Could you check a few things on this model? Use its own coordinates, in mm. Face numbers are marked on the shaded views. A direction names the side the tool comes from. Coordinates: 2 decimals unless noted, no trailing zeros. Write each loop counter-clockwise with the first axis right and the second up, starting at its lowest first coordinate (ties: lowest second). Pieces come first, ordered by that corner, then holes.
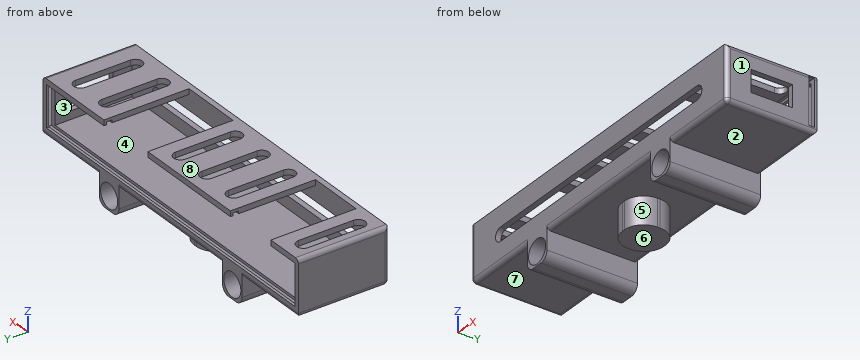
```python
from build123d import *

# Parameters (mm, degrees)
ESBO_O1_W                = 130
ESBO_O1_H                = 33
RESSALTO_EXTRUS_O1_DEPTH = 3
ESBO_O2_W                = 130
ESBO_O2_H                = 33
ESBO_O2_W_2              = 126
ESBO_O2_H_2              = 29
EXTRUS_O_FINA1_DEPTH     = 17
ESBO_O3_W                = 126.5
ESBO_O3_H                = 15
CORTE_EXTRUS_O1_DEPTH    = 2
ESBO_O4_W                = 8
ESBO_O4_H                = 15
CORTE_EXTRUS_O2_DEPTH    = 2
ESBO_O7_W                = 42
ESBO_O7_H                = 2
ESBO_O7_W_2              = 12
ESBO_O7_W_3              = 29
RESSALTO_EXTRUS_O2_DEPTH = 29
ESBO_O8_W                = 20.6
ESBO_O8_H                = 2
ESBO_O8_W_2              = 22.4
CORTE_EXTRUS_O4_DEPTH    = 2
CORTE_EXTRUS_O3_REACH    = 134.56
ESBO_O5_W                = 17
ESBO_O5_H                = 2
CORTE_EXTRUS_O5_DEPTH    = 2
CORTE_EXTRUS_O6_DEPTH    = 2
ESBO_O11_W               = 10
ESBO_O11_H               = 33
RESSALTO_EXTRUS_O3_DEPTH = 10
ESBO_O12_R               = 4.35
CORTE_EXTRUS_O7_DEPTH    = 76.591004756
ESBO_O13_W               = 15
ESBO_O13_H               = 15
RESSALTO_EXTRUS_O4_DEPTH = 10
FILETE1_R                = 7
FILETE2_R                = 3
FILETE3_R                = 1.5


with BuildPart() as part:
    # Esboço1 → Ressalto-extrusão1 (new body)
    with BuildSketch(Plane.XY):
        Rectangle(ESBO_O1_W, ESBO_O1_H)
    extrude(amount=RESSALTO_EXTRUS_O1_DEPTH)

    # Esboço2 → Extrusão-Fina1 (add)
    with BuildSketch(Plane.XY.offset(3)):
        Rectangle(ESBO_O2_W, ESBO_O2_H)
        Rectangle(ESBO_O2_W_2, ESBO_O2_H_2, mode=Mode.SUBTRACT)
    extrude(amount=EXTRUS_O_FINA1_DEPTH)

    # Esboço3 → Corte-extrusão1 (cut)
    with BuildSketch(Plane(origin=(0, 16.5, 0), x_dir=(1, 0, 0), z_dir=(0, 1, 0))):
        with Locations((0, -10.5)):
            Rectangle(ESBO_O3_W, ESBO_O3_H)
    extrude(amount=-CORTE_EXTRUS_O1_DEPTH, mode=Mode.SUBTRACT)

    # Esboço4 → Corte-extrusão2 (cut)
    with BuildSketch(Plane(origin=(65, 0, 0), x_dir=(0, 0, -1), z_dir=(1, 0, 0))):
        with Locations((-10, 0)):
            Rectangle(ESBO_O4_W, ESBO_O4_H)
    extrude(amount=-CORTE_EXTRUS_O2_DEPTH, mode=Mode.SUBTRACT)

    # Esboço7 → Ressalto-extrusão2 (add)
    with BuildSketch(Plane(origin=(0, -14.5, 0), x_dir=(1, 0, 0), z_dir=(0, 1, 0))):
        with Locations((-9.4, -19)):
            Rectangle(ESBO_O7_W, ESBO_O7_H)
        with Locations((-57, -19)):
            Rectangle(ESBO_O7_W_2, ESBO_O7_H)
        with Locations((48.5, -19)):
            Rectangle(ESBO_O7_W_3, ESBO_O7_H)
    extrude(amount=RESSALTO_EXTRUS_O2_DEPTH)

    # Esboço8 → Corte-extrusão4 (cut)
    with BuildSketch(Plane(origin=(0, 16.5, 0), x_dir=(1, 0, 0), z_dir=(0, 1, 0))):
        with Locations((-40.7, -19)):
            Rectangle(ESBO_O8_W, ESBO_O8_H)
        with Locations((22.8, -19)):
            Rectangle(ESBO_O8_W_2, ESBO_O8_H)
    extrude(amount=-CORTE_EXTRUS_O4_DEPTH, mode=Mode.SUBTRACT)

    # Corte-extrusão3: up to this face of the body (flat: up to its plane)
    corte_extrus_o3_end = Plane(part.part.faces().sort_by_distance((-63.25, 15.5, 10.5))[0])
    # Esboço5 → Corte-extrusão3 (cut, up to the picked face)
    with BuildSketch(Plane(origin=(65, 0, 0), x_dir=(0, 0, -1), z_dir=(1, 0, 0)), mode=Mode.PRIVATE) as corte_extrus_o3_sk1:
        with Locations((-10.5, 14.5)):
            Rectangle(ESBO_O5_W, ESBO_O5_H)
    corte_extrus_o3_tool1 = split(extrude(corte_extrus_o3_sk1.sketch, amount=-CORTE_EXTRUS_O3_REACH, mode=Mode.PRIVATE), bisect_by=corte_extrus_o3_end, keep=Keep.BOTH, mode=Mode.PRIVATE)
    add(corte_extrus_o3_tool1.solids().sort_by(Axis((65, 14.5, 10.5), (-1, 0, 0)))[0], mode=Mode.SUBTRACT)

    # Esboço9 → Corte-extrusão5 (cut)
    with BuildSketch(Plane.XY.offset(20)):
        with BuildLine():
            Line((-61, -10), (-61, 10))
            ThreePointArc((-61, 10), (-58.5, 12.5), (-56, 10))
            Line((-56, 10), (-56, -10))
            ThreePointArc((-56, -10), (-58.5, -12.5), (-61, -10))
        make_face()
        with BuildLine():
            Line((-25.4, -10), (-25.4, 10))
            ThreePointArc((-25.4, 10), (-22.9, 12.5), (-20.4, 10))
            Line((-20.4, 10), (-20.4, -10))
            ThreePointArc((-20.4, -10), (-22.9, -12.5), (-25.4, -10))
        make_face()
        with BuildLine():
            Line((-11.9, -10), (-11.9, 10))
            ThreePointArc((-11.9, 10), (-9.4, 12.5), (-6.9, 10))
            Line((-6.9, 10), (-6.9, -10))
            ThreePointArc((-6.9, -10), (-9.4, -12.5), (-11.9, -10))
        make_face()
        with BuildLine():
            Line((1.6, -10), (1.6, 10))
            ThreePointArc((1.6, 10), (4.1, 12.5), (6.6, 10))
            Line((6.6, 10), (6.6, -10))
            ThreePointArc((6.6, -10), (4.1, -12.5), (1.6, -10))
        make_face()
        with BuildLine():
            Line((39, -10), (39, 10))
            ThreePointArc((39, 10), (41.5, 12.5), (44, 10))
            Line((44, 10), (44, -10))
            ThreePointArc((44, -10), (41.5, -12.5), (39, -10))
        make_face()
        with BuildLine():
            Line((52.5, -10), (52.5, 10))
            ThreePointArc((52.5, 10), (55, 12.5), (57.5, 10))
            Line((57.5, 10), (57.5, -10))
            ThreePointArc((57.5, -10), (55, -12.5), (52.5, -10))
        make_face()
    extrude(amount=-CORTE_EXTRUS_O5_DEPTH, mode=Mode.SUBTRACT)

    # Esboço10 → Corte-extrusão6 (cut)
    with BuildSketch(Plane.XZ.offset(16.5)):
        with BuildLine():
            Line((-50, 12.5), (50, 12.5))
            ThreePointArc((50, 12.5), (52.5, 10), (50, 7.5))
            Line((50, 7.5), (-50, 7.5))
            ThreePointArc((-50, 7.5), (-52.5, 10), (-50, 12.5))
        make_face()
    extrude(amount=-CORTE_EXTRUS_O6_DEPTH, mode=Mode.SUBTRACT)

    # Esboço11 → Ressalto-extrusão3 (add)
    with BuildSketch(Plane(origin=(0, 0, 0), x_dir=(-1, 0, 0), z_dir=(0, 0, -1))):
        with Locations((-31.35, 0)):
            Rectangle(ESBO_O11_W, ESBO_O11_H)
        with Locations((31.35, 0)):
            Rectangle(ESBO_O11_W, ESBO_O11_H)
    extrude(amount=RESSALTO_EXTRUS_O3_DEPTH)

    # Esboço12 → Corte-extrusão7 (cut, through all)
    with BuildSketch(Plane.XZ.offset(16.5)):
        with Locations(Location((-31.35, -5, 0), (0, 0, 270))):
            Circle(ESBO_O12_R)
        with Locations(Location((31.35, -5, 0), (0, 0, 90))):
            Circle(ESBO_O12_R)
    extrude(amount=-CORTE_EXTRUS_O7_DEPTH, mode=Mode.SUBTRACT)

    # Esboço13 → Ressalto-extrusão4 (add)
    with BuildSketch(Plane(origin=(0, 0, 0), x_dir=(-1, 0, 0), z_dir=(0, 0, -1))):
        Rectangle(ESBO_O13_W, ESBO_O13_H)
    extrude(amount=RESSALTO_EXTRUS_O4_DEPTH)

    # Filete1
    filete1_edges = [part.edges().sort_by_distance(p)[0] for p in [
        (-7.5, -7.5, -5),
        (-7.5, 7.5, -5),
        (7.5, 7.5, -5),
        (7.5, -7.5, -5),
    ]]
    fillet(filete1_edges, radius=FILETE1_R)

    # Filete2
    filete2_edges = [part.edges().sort_by_distance(p)[0] for p in [
        (26.35, 0, -10),
        (36.35, 0, -10),
        (-36.35, 0, -10),
        (-26.35, 0, -10),
    ]]
    fillet(filete2_edges, radius=FILETE2_R)

    # Filete3
    # the kernel refuses this fillet: 1.5 mm, written as the material it takes off along each edge
    with BuildSketch(Plane(origin=(63.5, -15, 1.5), x_dir=(0, -1, 0), z_dir=(1, 0, 0))) as filete3_piece_1_section:
        Polygon((0, 0), (FILETE3_R, 0), (FILETE3_R, FILETE3_R), (0, FILETE3_R), align=None)
    filete3_piece_1 = extrude(amount=FILETE3_R, mode=Mode.PRIVATE)
    filete3_piece_1 = filete3_piece_1 - Plane(origin=(63.5, -15, 1.5), x_dir=(0, 0.7071067811865475, 0.7071067811865475), z_dir=(1, 0, 0)) * Sphere(FILETE3_R, mode=Mode.PRIVATE)
    add(filete3_piece_1, mode=Mode.SUBTRACT)
    with BuildSketch(Plane(origin=(-63.5, -15, 1.5), x_dir=(0, -1, 0), z_dir=(-1, 0, 0))) as filete3_piece_2_section:
        Polygon((0, 0), (FILETE3_R, 0), (FILETE3_R, -FILETE3_R), (0, -FILETE3_R), align=None)
    filete3_piece_2 = extrude(amount=FILETE3_R, mode=Mode.PRIVATE)
    filete3_piece_2 = filete3_piece_2 - Plane(origin=(-63.5, -15, 1.5), x_dir=(0, 0.7071067811865475, 0.7071067811865475), z_dir=(-1, 0, 0)) * Sphere(FILETE3_R, mode=Mode.PRIVATE)
    add(filete3_piece_2, mode=Mode.SUBTRACT)
    with BuildSketch(Plane(origin=(68.75, 16.5, 0), x_dir=(0, 0, 1), z_dir=(-1, 0, 0)), Plane(origin=(-36.35, 16.5, 0), x_dir=(0, 0, 1), z_dir=(-1, 0, 0))) as filete3_piece_3:
        with BuildLine():
            CenterArc((FILETE3_R, -FILETE3_R), FILETE3_R, 90, 90)
            Line((0, -FILETE3_R), (0, 0))
            Line((0, 0), (FILETE3_R, 0))
        make_face()
    extrude(amount=32.4, mode=Mode.SUBTRACT)
    with BuildSketch(Plane(origin=(26.35, 16.5, 0), x_dir=(0, 0, 1), z_dir=(-1, 0, 0))) as filete3_piece_4:
        with BuildLine():
            CenterArc((FILETE3_R, -FILETE3_R), FILETE3_R, 90, 90)
            Line((0, -FILETE3_R), (0, 0))
            Line((0, 0), (FILETE3_R, 0))
        make_face()
    extrude(amount=52.7, mode=Mode.SUBTRACT)
    with BuildSketch(Plane(origin=(65, -15, 0), x_dir=(-1, 0, 0), z_dir=(0, 1, 0)), Plane(origin=(-65, 20.25, 0), x_dir=(1, 0, 0), z_dir=(0, -1, 0))) as filete3_piece_5:
        with BuildLine():
            CenterArc((FILETE3_R, FILETE3_R), FILETE3_R, 180, 90)
            Line((0, FILETE3_R), (0, 0))
            Line((0, 0), (FILETE3_R, 0))
        make_face()
    extrude(amount=35.25, mode=Mode.SUBTRACT)
    with BuildSketch(Plane(origin=(65, -16.5, 1.5), x_dir=(-1, 0, 0), z_dir=(0, 0, 1)), Plane(origin=(-65, -16.5, 23.75), x_dir=(1, 0, 0), z_dir=(0, 0, -1))) as filete3_piece_6:
        with BuildLine():
            CenterArc((FILETE3_R, -FILETE3_R), FILETE3_R, 90, 90)
            Line((0, -FILETE3_R), (0, 0))
            Line((0, 0), (FILETE3_R, 0))
        make_face()
    extrude(amount=22.25, mode=Mode.SUBTRACT)
    with BuildSketch(Plane(origin=(65, -20.25, 20), x_dir=(0, 0, -1), z_dir=(0, 1, 0))) as filete3_piece_7:
        with BuildLine():
            CenterArc((FILETE3_R, FILETE3_R), FILETE3_R, 180, 90)
            Line((0, FILETE3_R), (0, 0))
            Line((0, 0), (FILETE3_R, 0))
        make_face()
    extrude(amount=40.5, mode=Mode.SUBTRACT)
    with BuildSketch(Plane(origin=(-65, 20.25, 20), x_dir=(1, 0, 0), z_dir=(0, -1, 0))) as filete3_piece_8:
        with BuildLine():
            CenterArc((FILETE3_R, -FILETE3_R), FILETE3_R, 90, 90)
            Line((0, -FILETE3_R), (0, 0))
            Line((0, 0), (FILETE3_R, 0))
        make_face()
    extrude(amount=40.5, mode=Mode.SUBTRACT)
    with BuildSketch(Plane(origin=(36.35, -16.5, 0), x_dir=(0, 0, 1), z_dir=(1, 0, 0)), Plane(origin=(-63.5, -16.5, 0), x_dir=(0, 0, 1), z_dir=(1, 0, 0))) as filete3_piece_9:
        with BuildLine():
            CenterArc((FILETE3_R, -FILETE3_R), FILETE3_R, 90, 90)
            Line((0, -FILETE3_R), (0, 0))
            Line((0, 0), (FILETE3_R, 0))
        make_face()
    extrude(amount=27.15, mode=Mode.SUBTRACT)
    with BuildSketch(Plane(origin=(-26.35, -16.5, 0), x_dir=(0, 1, 0), z_dir=(1, 0, 0))) as filete3_piece_10:
        with BuildLine():
            CenterArc((FILETE3_R, FILETE3_R), FILETE3_R, 180, 90)
            Line((0, FILETE3_R), (0, 0))
            Line((0, 0), (FILETE3_R, 0))
        make_face()
    extrude(amount=52.7, mode=Mode.SUBTRACT)


solid = part.part
```
1. Please list where these lines run through material, in increasing order: line 1 along Z through (x, y) = (-31, -2); line 2 along X through (y, z) = (-0.5, -5); line 3 along X through (y, z) = (-0.5, 15).
Verdict:
line 1: z = -10 to -9.34, -0.66 to 3
line 2: x = -36.35 to -35.7, -27 to -26.35, -7.5 to 7.5, 26.35 to 27, 35.7 to 36.35
line 3: x = -65 to -63, 63 to 65
2. On a 3-axis mill with a long thin cutter (end or side, diameter ignored), from which of +Z, -Z, +X, -X, +Y, -Y can I reach the whole of each face in a straight line? I mean the marked faces 4, 5, 6, 7 and 8. Say none if no direction works.
Verdict:
face 4: +Y
face 5: -Z, -Y
face 6: -Z, +X, -X, +Y, -Y
face 7: -Z, -X, +Y, -Y
face 8: +Z, +X, -X, +Y, -Y
3. I want a section at A-A on x = 31.35. Please give me the cut outline in (y, z), plus the area to 3 significant figures.
Verdict:
outline: (-16.5, -10) - (16.5, -10) - (16.5, -9.35) - (-16.5, -9.35) - close; (-16.5, -0.65) - (16.5, -0.65) - (16.5, 3) - (15.5, 3) - (15.5, 2) - (13.5, 2) - (13.5, 3) - (-14.5, 3) - (-14.5, 7.5) - (-16.5, 7.5) - close; (-16.5, 12.5) - (-14.5, 12.5) - (-14.5, 20) - (-16.5, 20) - close
area: 164 mm2
4. If we mould it in two halves opening along X, with no side actions, what happens to the marked faces 1, 2 and 3? For each: pulls with the +X half, pulls with the -X half, needs draft (parallel to the pull), parting line crosses it, or undercut.
Verdict:
face 1: pulls with the +X half
face 2: needs draft
face 3: undercut
5. For pin 1 (1.1 mm diameter, centred on y = 0, z = -4.5, fed in from +X); pin 2 (1.5 mm diameter, centred on x = -8.5, y = -3.5, fed in from +Z); pin 3 (1.6 mm diameter, centred on y = -1, z = 19.5, fed in from -X), each with a flat end and sliding along its axis, tell me the tip position at first contact or that it passes through.
Verdict:
pin 1: stops at x = 36.35
pin 2: stops at z = 3
pin 3: stops at x = -64.99
6. I want a section at D-D on z = 16.75. Please give me the cut outline in (x, y).
Verdict:
outline: (-65, -15) arc R1.5 ccw to (-63.5, -16.5) - (63.5, -16.5) arc R1.5 ccw to (65, -15) - (65, 13.5) - (63, 13.5) - (63, -14.5) - (-63, -14.5) - (-63, 13.5) - (-63.25, 13.5) - (-63.25, 16.5) - (-65, 16.5) - close; (63.25, 15.5) - (65, 15.5) - (65, 16.5) - (63.25, 16.5) - close
7. I want a section at C-C on x = 55. Please give me the cut outline in (y, z), plus the area to 3 significant figures.
Verdict:
outline: (-16.5, 1.5) arc R1.5 ccw to (-15, 0) - (15, 0) arc R1.5 ccw to (16.5, 1.5) - (16.5, 3) - (15.5, 3) - (15.5, 2) - (13.5, 2) - (13.5, 3) - (-14.5, 3) - (-14.5, 18) - (-12.5, 18) - (-12.5, 20) - (-16.5, 20) - close; (12.5, 18) - (13.5, 18) - (13.5, 19) - (15.5, 19) - (15.5, 18) - (16.5, 18) - (16.5, 20) - (12.5, 20) - close
area: 140 mm2
8. I want a section at B-B on z = -5. Please give me the cut outline in (x, y), plus the area to 3 significant figures.
Verdict:
outline: (-36.35, -16.5) - (-35.7, -16.5) - (-35.7, 16.5) - (-36.35, 16.5) - close; (-27, -16.5) - (-26.35, -16.5) - (-26.35, 16.5) - (-27, 16.5) - close; (-7.5, -0.5) arc R7 ccw to (-0.5, -7.5) - (0.5, -7.5) arc R7 ccw to (7.5, -0.5) - (7.5, 0.5) arc R7 ccw to (0.5, 7.5) - (-0.5, 7.5) arc R7 ccw to (-7.5, 0.5) - close; (26.35, -16.5) - (27, -16.5) - (27, 16.5) - (26.35, 16.5) - close; (35.7, -16.5) - (36.35, -16.5) - (36.35, 16.5) - (35.7, 16.5) - close
area: 269 mm2
